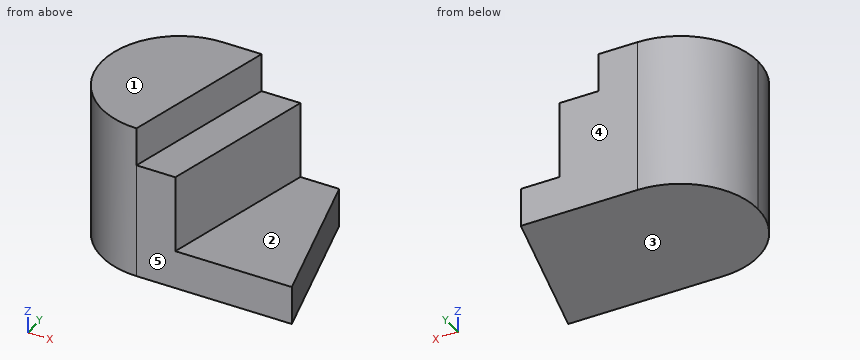
```python
from build123d import *

# Parameters (mm, degrees)
F0_W     = 60
F0_H     = 40
F1_DEPTH = 40
F2_R     = 19.99999
F4_DEPTH = 40
F6_DEPTH = 30
F8_DEPTH = 10


# Not quite as in the source:
# - a fillet or chamfer is up to 0.001 mm smaller than in the source, because OpenCascade refuses the exact size


with BuildPart() as f1:
    # F0 (on Top) → F1 (new body)
    with BuildSketch(Plane.XY):
        with Locations((30, 20)):
            Rectangle(F0_W, F0_H)
    extrude(amount=F1_DEPTH)

    # F2 (radius 20 in the source; OpenCascade refuses exactly that, so slightly less here)
    f2_edges = [f1.edges().sort_by_distance(p)[0] for p in [
        (0, 40, 20),
        (0, 0, 20),
    ]]
    fillet(f2_edges, radius=F2_R)

    # F3 (on face) → F4 (cut)
    with BuildSketch(Plane.XY.offset(40)):
        Polygon((60, 0), (60, 40), (50, 40), align=None)
    extrude(amount=-F4_DEPTH, mode=Mode.SUBTRACT)

    # F5 (on face) → F6 (cut)
    with BuildSketch(Plane.XY.offset(40)):
        Polygon((60, 0), (50, 40), (40, 40), (30, 0), align=None)
    extrude(amount=-F6_DEPTH, mode=Mode.SUBTRACT)

    # F7 (on face) → F8 (cut)
    with BuildSketch(Plane.XY.offset(40)):
        Polygon((30, 0), (40, 40), (30, 40), (20, 0), align=None)
    extrude(amount=-F8_DEPTH, mode=Mode.SUBTRACT)


solid = f1.part
```
For this review, take the finished solid that the model builds, in its own axes (mm). Face numbers are marked on the shaded views. A direction names the side the tool comes from. Round coordinates to 2 decimals unless told otherwise and drop trailing zeros. Write each loop counter-clockwise with the first axis right and the second up, starting at its lowest first coordinate (ties: lowest second). Pieces come first, ordered by that corner, then holes. Notation, with made-up numbers: (86.5, 12) - (93.5, 12) arc R25 ccw to (93.5, 51) - close; hole circle Ø11 at (-37, -17). An arc over 180 degrees is marked (long way). Answer as a JSON object with one key per item and string values.
1. Tool access review of the marked faces 1 and 2: name each direction out of +Z, -Z, +X, -X, +Y, -Y from which nothing blocks a thin tool from reaching the whole face with its end or side.
Response values:
{"face 1": "+Z, +X, -X, +Y, -Y", "face 2": "+Z, +X, -Y"}
2. We need section B-B on y = 28. Give the boundary of the cut face in (x, z), then the cut area to 3 significant figures.
Response values:
{"outline": "(1.67, 0) - (53, 0) - (53, 10) - (37, 10) - (37, 30) - (27, 30) - (27, 40) - (1.67, 40) - close", "area": "1,470 mm2"}
3. Draft analysis for pull direction Y (two halves, no side actions). For the marked faces 3, 4 and 5, state which applies: +Y half, -Y half, draft (parallel to the pull), parting line (faces both ways), or undercut.
Response values:
{"face 3": "draft", "face 4": "+Y half", "face 5": "-Y half"}
4. To check wall thickness, follow line 1 along Z through (x, y) = (52.5, 17); line 2 along Z through (x, y) = (23, 11); line 3 along X through (y, z) = (23.5, 12.5) (3 decimals). State the ranges of each line that lie inside material, in increasing order.
Response values:
{"line 1": "z = 0 to 10", "line 2": "z = 0 to 30", "line 3": "x = 0.309 to 35.875"}
5. We need section D-D on y = 12. Give the boundary of the cut face in (x, z).
Response values:
{"outline": "(1.67, 0) - (57, 0) - (57, 10) - (33, 10) - (33, 30) - (23, 30) - (23, 40) - (1.67, 40) - close"}
6. We need section A-A on x = 28.5. Give the boundary of the cut face in (y, z).
Response values:
{"outline": "(0, 0) - (40, 0) - (40, 40) - (34, 40) - (34, 30) - (0, 30) - close"}
7. For pin 1 Ø6 at (y, z) = (11.5, 23) entering from -X; pin 2 Ø6 at (x, z) = (14.5, 35) entering from -Y; pin 3 Ø3 at (y, z) = (28.5, 10) entering from -X (3 decimals), all flat-tipped, find the tip position at first contact; note any pin that passes through.
Response values:
{"pin 1": "stops at x = 0.77", "pin 2": "stops at y = 0.16", "pin 3": "stops at x = 1.265"}
